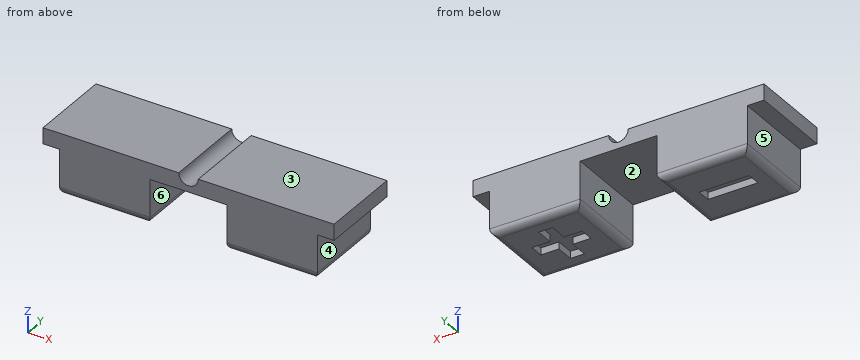
```python
from build123d import *

# Parameters (mm, degrees)
EXTRUDE_1_DEPTH     = 6
SKETCH_2_W          = 1.8
SKETCH_2_H          = 0.5
SKETCH_2_W_2        = 1
SKETCH_2_H_2        = 1.3
SKETCH_2_W_3        = 1.3
SKETCH_2_W_4        = 0.5
CUT_EXTRUDE_1_DEPTH = 0.5
FILLET_1_R          = 0.5


with BuildPart() as part:
    # 草图1 → 凸台-拉伸1 (new body)
    with BuildSketch(Plane(origin=(0, 0, 0), x_dir=(1, 0, 0), z_dir=(0, 1, 0))):
        with BuildLine():
            Line((-153.747698535, 92.341311307), (-153.747698535, 90.141311307))
            Line((-153.747698535, 90.141311307), (-154.947698535, 90.141311307))
            Line((-154.947698535, 90.141311307), (-154.947698535, 89.341311307))
            Line((-154.947698535, 89.341311307), (-154.947698535, 88.991311307))
            Line((-154.947698535, 88.991311307), (-145.197698535, 88.991311307))
            ThreePointArc((-145.197698535, 88.991311307), (-144.497698535, 89.691311307), (-143.797698535, 88.991311307))
            Line((-143.797698535, 88.991311307), (-134.047698535, 88.991311307))
            Line((-134.047698535, 88.991311307), (-134.047698535, 89.341311307))
            Line((-134.047698535, 89.341311307), (-134.047698535, 90.141311307))
            Line((-134.047698535, 90.141311307), (-135.247698535, 90.141311307))
            Line((-135.247698535, 90.141311307), (-135.247698535, 93.341311307))
            Line((-135.247698535, 93.341311307), (-141.747698535, 93.341311307))
            Line((-141.747698535, 93.341311307), (-141.747698535, 90.141311307))
            Line((-141.747698535, 90.141311307), (-141.997698535, 90.141311307))
            Line((-141.997698535, 90.141311307), (-147.247698535, 90.141311307))
            Line((-147.247698535, 90.141311307), (-147.247698535, 93.341311307))
            Line((-147.247698535, 93.341311307), (-153.747698535, 93.341311307))
            Line((-153.747698535, 93.341311307), (-153.747698535, 92.341311307))
        make_face()
    extrude(amount=EXTRUDE_1_DEPTH)

    # 草图2 → 切除-拉伸1 (cut)
    with BuildSketch(Plane(origin=(0, 0, -93.341311307), x_dir=(-1, 0, 0), z_dir=(0, 0, -1))):
        Polygon((148.697698535, 3.5), (148.697698535, 3), (150.497698535, 3), (152.297698535, 3), (152.297698535, 3.5), align=None)
        with Locations((151.397698535, 2.75)):
            Rectangle(SKETCH_2_W, SKETCH_2_H)
        with Locations((149.597698535, 2.75)):
            Rectangle(SKETCH_2_W, SKETCH_2_H)
        with Locations((138.497698535, 4.15)):
            Rectangle(SKETCH_2_W_2, SKETCH_2_H_2)
        with Locations((137.347698535, 3.25)):
            Rectangle(SKETCH_2_W_3, SKETCH_2_H)
        Polygon((137.997698535, 3.5), (137.997698535, 3), (138.497698535, 3), (138.997698535, 3), (138.997698535, 3.5), align=None)
        with Locations((139.647698535, 3.25)):
            Rectangle(SKETCH_2_W_3, SKETCH_2_H)
        with Locations((139.647698535, 2.75)):
            Rectangle(SKETCH_2_W_3, SKETCH_2_H)
        with Locations((138.747698535, 2.75)):
            Rectangle(SKETCH_2_W_4, SKETCH_2_H)
        with Locations((138.247698535, 2.75)):
            Rectangle(SKETCH_2_W_4, SKETCH_2_H)
        with Locations((137.347698535, 2.75)):
            Rectangle(SKETCH_2_W_3, SKETCH_2_H)
        with Locations((138.247698535, 1.85)):
            Rectangle(SKETCH_2_W_4, SKETCH_2_H_2)
        with Locations((138.747698535, 1.85)):
            Rectangle(SKETCH_2_W_4, SKETCH_2_H_2)
    extrude(amount=-CUT_EXTRUDE_1_DEPTH, mode=Mode.SUBTRACT)

    # 圆角1
    fillet_1_edges = [part.edges().sort_by_distance(p)[0] for p in [
        (-150.497698535, 0, -93.341311307),
        (-138.497698535, 0, -93.341311307),
        (-138.497698535, 6, -93.341311307),
        (-153.747698535, 3, -93.341311307),
        (-147.247698535, 3, -93.341311307),
        (-141.747698535, 3, -93.341311307),
        (-135.247698535, 3, -93.341311307),
        (-150.497698535, 6, -93.341311307),
    ]]
    fillet(fillet_1_edges, radius=FILLET_1_R)


solid = part.part
```
Design review of the part built by this model. Coordinates are the model's own, in mm. Face numbers are marked on the shaded views. A direction names the side the tool comes from. Give positions to 0.01 mm unless a question says otherwise; leave off trailing zeros. Write each loop counter-clockwise with the first axis right and the second up, starting at its lowest first coordinate (ties: lowest second). Pieces come first, ordered by that corner, then holes. Notation, with made-up numbers: (36, 41.5) - (90, 41.5) arc R28 ccw to (90, 80.5) - close; hole circle Ø5 at (43.25, 42). An arc over 180 degrees is marked (long way). Return JSON: item names as keys, results as strings. Group by question number.
(1) To check wall thickness, follow probe 1 along X at (y, z) = (2.55, -92.65); probe 2 along X at (y, z) = (2.4, -92.95); probe 3 along Z at (x, y) = (-147, 5.55). State the ranges of each line that lie inside material, in increasing order.
(2) Insertion check: pin 1 (1.5 mm diameter, centred on y = 2, z = -91, fed in from +X); pin 2 (1 mm diameter, centred on x = -154.5, y = 3, fed in from -Z); pin 3 (0.5 mm diameter, centred on x = -150, y = 3, fed in from -Z). Each pin has a flat end and moves straight along its axis. Give the tip position at first contact, or say it passes through.
(3) We need section A-A, the plane z = -90.9. Give the boundary of the cut face in (x, y), then the cut area to 3 significant figures.
(4) Machinability: for the marked faces 4, 5 and 6, which of the approach directions +Z, -Z, +X, -X, +Y, -Y give a long, thin tool a straight path to every point of the face, cutting with its end or side? Answer none if there is none.
(5) We need section B-B, the plane x = -149.25. Give the boundary of the cut face in (y, z), then the cut area to 3 significant figures.
(6) We need section D-D, the plane z = -89.45. Give the boundary of the cut face in (x, y).
(7) We need section C-C, the plane y = 2.8. Give the boundary of the cut face in (x, z), then the cut area to 3 significant figures.
(8) Mouldability with a two-part tool opening along Z and no side actions: class the marked faces 1, 2 and 3 as +Z half, -Z half, draft (parallel to the pull), parting line (faces both ways), or undercut.
Reported:
{
 "1": {"probe 1": "x = -153.75 to -147.25, -141.75 to -135.25", "probe 2": "x = -153.74 to -147.26, -141.74 to -139, -138 to -135.26", "probe 3": "z = -90.14 to -88.99"},
 "2": {"pin 1": "stops at x = -135.25", "pin 2": "stops at z = -90.14", "pin 3": "stops at z = -92.84"},
 "3": {"outline": "(-153.75, 0) - (-147.25, 0) - (-147.25, 6) - (-153.75, 6) - close; (-141.75, 0) - (-135.25, 0) - (-135.25, 6) - (-141.75, 6) - close", "area": "78.0 mm2"},
 "4": {"face 4": "-Z, +X, +Y, -Y", "face 5": "-Z, -X, +Y, -Y", "face 6": "-Z, +Y, -Y"},
 "5": {"outline": "(0, -92.84) arc R0.5 ccw to (0.5, -93.34) - (2.5, -93.34) - (2.5, -92.84) - (3.5, -92.84) - (3.5, -93.34) - (5.5, -93.34) arc R0.5 ccw to (6, -92.84) - (6, -88.99) - (0, -88.99) - close", "area": "25.5 mm2"},
 "6": {"outline": "(-154.95, 0) - (-145.03, 0) - (-145.03, 6) - (-154.95, 6) - close; (-143.97, 0) - (-134.05, 0) - (-134.05, 6) - (-143.97, 6) - close"},
 "7": {"outline": "(-154.95, -90.14) - (-153.75, -90.14) - (-153.75, -92.84) arc R0.5 ccw to (-153.25, -93.34) - (-152.3, -93.34) - (-152.3, -92.84) - (-148.7, -92.84) - (-148.7, -93.34) - (-147.75, -93.34) arc R0.5 ccw to (-147.25, -92.84) - (-147.25, -90.14) - (-141.75, -90.14) - (-141.75, -92.84) arc R0.5 ccw to (-141.25, -93.34) - (-140.3, -93.34) - (-140.3, -92.84) - (-136.7, -92.84) - (-136.7, -93.34) - (-135.75, -93.34) arc R0.5 ccw to (-135.25, -92.84) - (-135.25, -90.14) - (-134.05, -90.14) - (-134.05, -88.99) - (-143.8, -88.99) arc R0.7 cw to (-145.2, -88.99) - (-154.95, -88.99) - close", "area": "61.1 mm2"},
 "8": {"face 1": "draft", "face 2": "-Z half", "face 3": "+Z half"}
}
